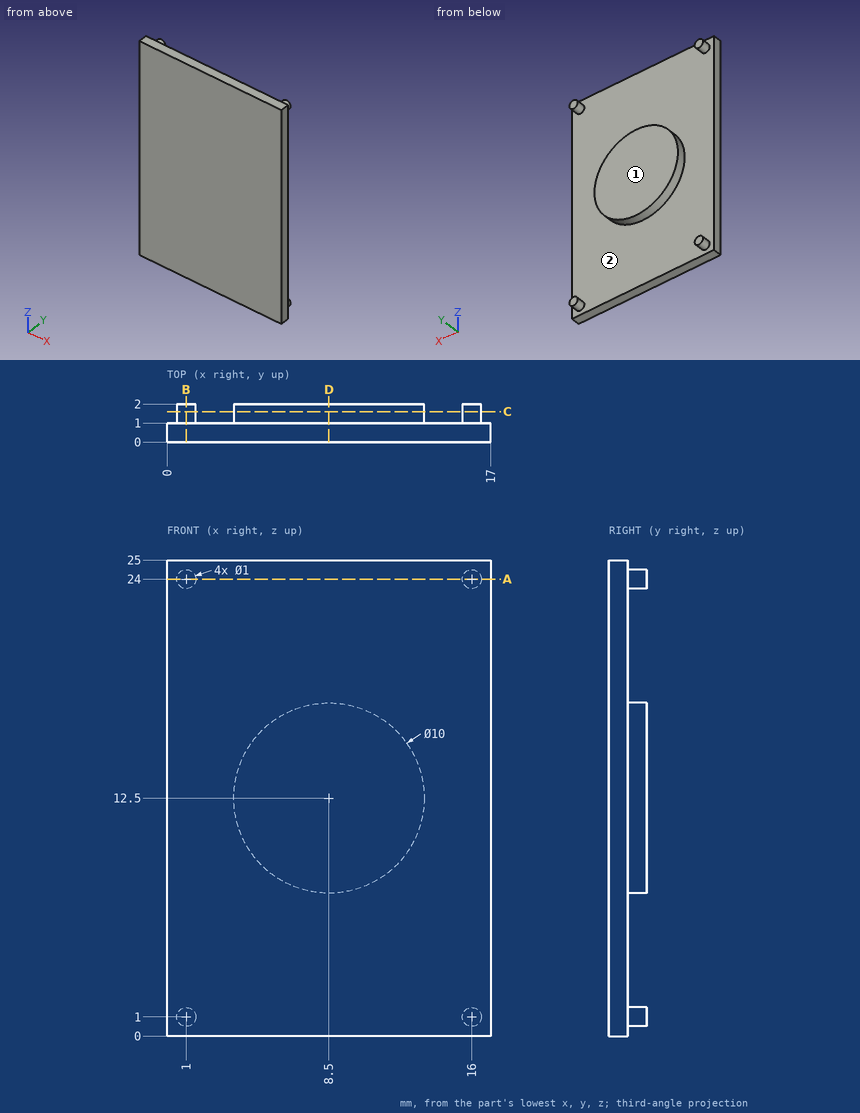
Check sheet for the drawn part. Datum: minimum x, y, z corner. Units: mm. A direction names the side the tool comes from. Give positions to 0.01 mm unless a question says otherwise; leave off trailing zeros. Order: outer loops, then holes, each group sorted by start corner. A loop starts at its lowest first (then second) coordinate and runs counter-clockwise, first axis right, second up. Notation, with made-up numbers: (-35, 7) - (-5, 7) arc R25 ccw to (-5, 34) - close; hole circle Ø9 at (-35.5, 4.5). An arc over 180 degrees is marked (long way). Write item = value, one per line. Start each with the question number.
1) Section check A-A (z = 24). Enter the section's corners in (x, y).
2) Section check B-B (x = 1). Enter the section's corners in (y, z).
3) Scan lines: L1, parallel to Y at x = 13, z = 4.75; L2, parallel to X at y = 1.1, z = 12.5; L3, parallel to Z at x = 9.5, y = 1.55. Record each from-to range of solid material in increasing order.
4) Access from +Z, -Z, +X, -X, +Y, -Y to the whole of each face (thin tool, end or side, straight path). Record for the marked faces 1 and 2.
5) Section check D-D (x = 8.5). Enter the section's corners in (y, z), then the cut area to 3 significant figures.
6) Section check C-C (y = 1.6). Enter the section's corners in (x, z).
Geometry check:
q1.outline = (0, 0) - (17, 0) - (17, 1) - (16.5, 1) - (16.5, 2) - (15.5, 2) - (15.5, 1) - (1.5, 1) - (1.5, 2) - (0.5, 2) - (0.5, 1) - (0, 1) - close
q2.outline = (0, 0) - (1, 0) - (1, 0.5) - (2, 0.5) - (2, 1.5) - (1, 1.5) - (1, 23.5) - (2, 23.5) - (2, 24.5) - (1, 24.5) - (1, 25) - (0, 25) - close
q3.L1 = 0 to 1
q3.L2 = 3.5 to 13.5
q3.L3 = 7.6 to 17.4
q4.face_1 = +Z, -Z, +X, -X, +Y
q4.face_2 = +Y
q5.outline = (0, 0) - (1, 0) - (1, 7.5) - (2, 7.5) - (2, 17.5) - (1, 17.5) - (1, 25) - (0, 25) - close
q5.area = 35.0 mm2
q6.outline = circle Ø1 at (1, 1); circle Ø1 at (1, 24); circle Ø10 at (8.5, 12.5); circle Ø1 at (16, 1); circle Ø1 at (16, 24)
